Here's how the part is built. I have some questions about the finished solid (model axes, mm). Face numbers are marked on the shaded views. A direction names the side the tool comes from. Coordinates: 2 decimals unless noted, no trailing zeros. Loops run counter-clockwise (first coordinate to the right, second up) from the corner with the lowest first, then second, coordinate; pieces in that order, holes last. Notation, with made-up numbers: M 0.5,30.25 L 59.5,30.25 A15 cw 59.5,49.25 Z; hole C 62,14 d3. An arc over 180 degrees is marked long. Use one line per item in the form item = value. Start each with the question number.
(1) On a 3-axis mill with a long thin cutter (end or side, diameter ignored), from which of +Z, -Z, +X, -X, +Y, -Y can I reach the whole of each face in a straight line? I mean the marked faces 5 and 6. Say none if no direction works.
(2) Imagine slicing it at A-A, the plane y = -1.5. Please give me the cut outline in (x, z), and give its area (3 significant figures).
(3) Imagine slicing it at C-C, the plane y = -8.5. Please give me the cut outline in (x, z).
(4) Thinking about a two-plate mould opening in X: for the marked faces 1, 2, 3 and 4, which applies, +X half, -X half, draft (parallel to the pull), parting line (faces both ways), or undercut?
(5) Imagine slicing it at B-B, the plane z = 50. Please give me the cut outline in (x, y), and give its area (3 significant figures).
(6) Will these pins go through, and if not, where does the flat tip stop? P1, Ø5, axis at x = 14.5, y = -7, coming from the +Z side; P2, Ø8, axis at y = -10, z = 50, coming from the +X side; P3, Ø12, axis at y = -4.5, z = 11, coming from the +X side; P4, Ø11, axis at x = 14, y = -7, coming from the -Z side.
(7) Please list where these lines run through material, in increasing order: L1, parallel to X at y = 0.75, z = 50.5; L2, parallel to Y at x = 87.5, z = 50; L3, parallel to Y at x = 9.5, z = 50.
(8) Imagine slicing it at D-D, the plane y = 7. Please give me the cut outline in (x, z), and give its area (3 significant figures).
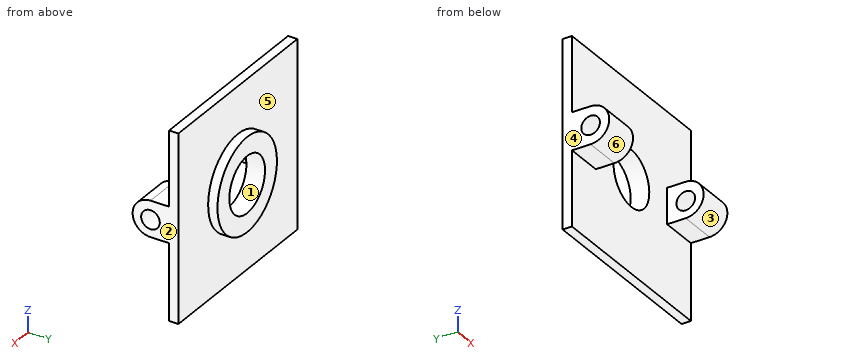
```python
from build123d import *

# Parameters (mm, degrees)
SKETCH_1_W          = 100
SKETCH_1_H          = 100
EXTRUDE_1_DEPTH     = 5
SKETCH_2_R          = 25
EXTRUDE_2_DEPTH     = 5
SKETCH_3_R          = 15
CUT_EXTRUDE_1_DEPTH = 10
EXTRUDE_3_DEPTH     = 20
EXTRUDE_4_DEPTH     = 20
SKETCH_6_R          = 5
CUT_EXTRUDE_2_DEPTH = 100


with BuildPart() as part:
    # 草图1 → 凸台-拉伸1 (new body)
    with BuildSketch(Plane(origin=(0, 0, 0), x_dir=(1, 0, 0), z_dir=(0, 1, 0))):
        with Locations((50, -50)):
            Rectangle(SKETCH_1_W, SKETCH_1_H)
    extrude(amount=EXTRUDE_1_DEPTH)

    # 草图2 → 凸台-拉伸2 (add)
    with BuildSketch(Plane(origin=(0, 5, 0), x_dir=(1, 0, 0), z_dir=(0, 1, 0))):
        with Locations(Location((50, -50, 0), (0, 0, 270))):
            Circle(SKETCH_2_R)
    extrude(amount=EXTRUDE_2_DEPTH)

    # 草图3 → 切除-拉伸1 (cut)
    with BuildSketch(Plane(origin=(0, 10, 0), x_dir=(1, 0, 0), z_dir=(0, 1, 0))):
        with Locations(Location((50, -50, 0), (0, 0, 270))):
            Circle(SKETCH_3_R)
    extrude(amount=-CUT_EXTRUDE_1_DEPTH, mode=Mode.SUBTRACT)

    # 草图4 → 凸台-拉伸3 (add)
    with BuildSketch(Plane(origin=(100, 0, 0), x_dir=(0, 0, -1), z_dir=(1, 0, 0))):
        with BuildLine():
            Line((-60, 0), (-40.851510599, 0))
            Line((-40.851510599, 0), (-40.851510599, -10))
            ThreePointArc((-40.851510599, -10), (-50.4257553, -19.5742447), (-60, -10))
            Line((-60, -10), (-60, 0))
        make_face()
    extrude(amount=-EXTRUDE_3_DEPTH)

    # 草图5 → 凸台-拉伸4 (add)
    with BuildSketch(Plane.ZY):
        with BuildLine():
            Line((40, 0), (60, 0))
            Line((60, 0), (60, -10))
            ThreePointArc((60, -10), (50, -20), (40, -10))
            Line((40, -10), (40, 0))
        make_face()
    extrude(amount=-EXTRUDE_4_DEPTH)

    # 草图6 → 切除-拉伸2 (cut)
    with BuildSketch(Plane.ZY):
        with Locations((50, -10)):
            Circle(SKETCH_6_R)
    extrude(amount=-CUT_EXTRUDE_2_DEPTH, mode=Mode.SUBTRACT)


solid = part.part
```
Answer:
q1.face_5 = +Y
q1.face_6 = +X, -X, -Y
q2.outline = M 0,40 L 20,40 L 20,60 L 0,60 Z; M 80,40.85 L 100,40.85 L 100,60 L 80,60 Z
q2.area = 783 mm²
q3.outline = M 0,40 L 20,40 L 20,45.23 L 0,45.23 Z; M 0,54.77 L 20,54.77 L 20,60 L 0,60 Z; M 80,40.85 L 100,40.85 L 100,45.23 L 80,45.23 Z; M 80,54.77 L 100,54.77 L 100,60 L 80,60 Z
q4.face_1 = undercut
q4.face_2 = +X half
q4.face_3 = draft
q4.face_4 = -X half
q5.outline = M 0,-20 L 20,-20 L 20,-15 L 0,-15 Z; M 0,-5 L 20,-5 L 20,0 L 35,0 L 35,10 L 25,10 L 25,5 L 0,5 Z; M 65,0 L 80,0 L 80,-5 L 100,-5 L 100,5 L 75,5 L 75,10 L 65,10 Z; M 80,-19.56 L 100,-19.56 L 100,-15 L 80,-15 Z
q5.area = 841 mm²
q6.P1 = 60
q6.P2 = through
q6.P3 = 100
q6.P4 = 40
q7.L1 = 0 to 35.01, 64.99 to 100
q7.L2 = -19.56 to -15, -5 to 5
q7.L3 = -20 to -15, -5 to 5
q8.outline = C 50,50 d50; hole C 50,50 d30
q8.area = 1,260 mm²
